The model under review builds one solid part; all positions refer to its coordinate system, in mm. Coordinates: 2 decimals unless noted, no trailing zeros. Write each loop counter-clockwise with the first axis right and the second up, starting at its lowest first coordinate (ties: lowest second). Pieces come first, ordered by that corner, then holes. Notation, with made-up numbers: (52, 27.25) - (79, 27.25) arc R20 ccw to (79, 44.25) - close; hole circle Ø3 at (41, -14). An arc over 180 degrees is marked (long way). Return JSON: item names as keys, results as strings. Group by question number.
(1) We need section C-C on x = -75. State the section outline as (y, z) points (3 decimals).
(2) We need section A-A on x = 99. State the section outline as (y, z) points (3 decimals), then the cut area to 3 significant figures.
(3) To check wall thickness, follow L1, parallel to X at y = 72.5, z = 0.35; L2, parallel to X at y = 37.5, z = 0.65; L3, parallel to X at y = 28, z = 0.75. State the ranges of each line that lie inside material, in increasing order. Write a range as from..to.
(4) For pin 1 Ø4 at (x, y) = (-29, -17.5) entering from -Z, flat-tipped, find the tip position at first contact; note if it passes through.
(5) We need section B-B on z = 0.55. State the section outline as (x, y) points (3 decimals), then the cut area to 3 significant figures.
(6) Draft analysis for pull direction Y (two halves, no side actions). For faces 1 (the face through (139.255, -95.272, 1.565)), 2 (the face through (1, 17, 3.175)), 3 (the face through (-126.8, 79, 1.6)), state which applies: released by +Y, released by -Y, zero draft, split by the parting line, or undercut.
```python
from build123d import *

# Parameters (mm, degrees)
F0_R     = 3.175
F0_W     = 92.075
F0_H     = 57.15
F0_W_2   = 38.1
F0_H_2   = 19.05
F1_DEPTH = 3.175


with BuildPart() as f1:
    # F0 (on Top) → F1 (new body)
    with BuildSketch(Plane.XY):
        with BuildLine():
            Line((130.373917, 129.706656), (-123.626083, 129.706656))
            ThreePointArc((-123.626083, 129.706656), (-132.606339, 125.986912), (-136.326083, 117.006656))
            Line((-136.326083, 117.006656), (-136.326083, -86.193344))
            ThreePointArc((-136.326083, -86.193344), (-132.606339, -95.1736), (-123.626083, -98.893344))
            Line((-123.626083, -98.893344), (130.373917, -98.893344))
            ThreePointArc((130.373917, -98.893344), (139.354173, -95.1736), (143.073917, -86.193344))
            Line((143.073917, -86.193344), (143.073917, 117.006656))
            ThreePointArc((143.073917, 117.006656), (139.354173, 125.986912), (130.373917, 129.706656))
        make_face()
        with Locations((-106.163583, -60.793344)):
            Circle(F0_R, mode=Mode.SUBTRACT)
        with Locations((-39.488583, 56.681656)):
            Rectangle(F0_W, F0_H, mode=Mode.SUBTRACT)
        with Locations((-123.626083, 78.906656)):
            Circle(F0_R, mode=Mode.SUBTRACT)
        with Locations((111.323917, 34.456656)):
            Rectangle(F0_W_2, F0_H_2, mode=Mode.SUBTRACT)
        with Locations((89.098917, 56.681656)):
            Circle(F0_R, mode=Mode.SUBTRACT)
    extrude(amount=F1_DEPTH)


solid = f1.part
```
Ans:
{
 "1": {"outline": "(-98.893, 0) - (28.107, 0) - (28.107, 3.175) - (-98.893, 3.175) - close; (85.257, 0) - (129.707, 0) - (129.707, 3.175) - (85.257, 3.175) - close"},
 "2": {"outline": "(-98.893, 0) - (24.932, 0) - (24.932, 3.175) - (-98.893, 3.175) - close; (43.982, 0) - (129.707, 0) - (129.707, 3.175) - (43.982, 3.175) - close", "area": "665 mm²"},
 "3": {"L1": "-136.33..-85.53, 6.55..143.07", "L2": "-136.33..-85.53, 6.55..92.27, 130.37..143.07", "L3": "-136.33..92.27, 130.37..143.07"},
 "4": {"pin 1": "z = 0"},
 "5": {"outline": "(-136.326, -86.193) arc R12.7 ccw to (-123.626, -98.893) - (130.374, -98.893) arc R12.7 ccw to (143.074, -86.193) - (143.074, 117.007) arc R12.7 ccw to (130.374, 129.707) - (-123.626, 129.707) arc R12.7 ccw to (-136.326, 117.007) - close; hole circle Ø6.35 at (-123.626, 78.907); hole circle Ø6.35 at (-106.164, -60.793); hole (-85.526, 28.107) - (6.549, 28.107) - (6.549, 85.257) - (-85.526, 85.257) - close; hole circle Ø6.35 at (89.099, 56.682); hole (92.274, 24.932) - (130.374, 24.932) - (130.374, 43.982) - (92.274, 43.982) - close", "area": "57,600 mm²"},
 "6": {"face 1": "released by -Y", "face 2": "zero draft", "face 3": "undercut"}
}
